Autodesk Inventor part; units mm, degrees
ref_plane "YZ Plane" through (0, 0, 0) normal (1, 0, 0) x (0, 1, 0)
ref_plane "XZ Plane" through (0, 0, 0) normal (0, 1, 0) x (-1, 0, 0)
ref_plane "XY Plane" through (0, 0, 0) normal (0, 0, 1) x (1, 0, 0)
sketch "スケッチ2" plane through (0, 0, 0) normal (0, 1, 0) x (-1, 0, 0)
  circle A0 centre (0, 0) radius 2
  circle A1 centre (0, 0) radius 2.75
  circle A2 centre (0, 0) radius 3.5
  line L0 (3.2709, 0) -> (-4.3069, 0) construction
  line L1 (-3.5, -2.0207) -> (0, -4.0415)
  line L2 (-3.5, 0) -> (-3.5, -2.0207)
  line L3 (0, 3.4516) -> (0, -4.8702) construction
  line L4 (-3.5, 2.0207) -> (0, 4.0415)
  line L5 (-3.5, 0) -> (-3.5, 2.0207)
  line L6 (3.5, -2.0207) -> (0, -4.0415)
  line L7 (3.5, 0) -> (3.5, -2.0207)
  line L8 (3.5, 2.0207) -> (0, 4.0415)
  line L9 (3.5, 0) -> (3.5, 2.0207)
  dimension "d8" = 7
  dimension "d6" = 4
  dimension "d7" = 5.5
  dimension "d25" = 120
extrude "押し出し1" add sketch "スケッチ2" against normal blind 0.7 contours A1
extrude "押し出し2" add sketch "スケッチ2" along normal blind 2.1 contours A1 | A2 | L7 L6 A2 | A2 L8 L9 | A2 L4 L8 | L6 L1 A2 | A2 L5 L4 | L1 L2 A2
chamfer "面取り1" distance 0.2 angle 45 6 edges at (3.5, 1.05, -2.0207) (0, 1.05, -4.0415) (-3.5, 1.05, -2.0207) (-3.5, 1.05, 2.0207) (0, 1.05, 4.0415) (3.5, 1.05, 2.0207)
chamfer "面取り2" distance 0.2 angle 45 6 edges at (3.4134, 2.1, -1.9707) (0, 2.1, -3.9415) (-3.4134, 2.1, -1.9707) (-3.4134, 2.1, 1.9707) (0, 2.1, 3.9415) (3.4134, 2.1, 1.9707)
thread "ねじ1"
properties part number "S4-07-3W" material "ステンレス鋼 AISI 304"
Verification items for the finished model (mm, model axes). A direction names the side the tool comes from. Give positions to 0.01 mm unless a question says otherwise; leave off trailing zeros. Loops run counter-clockwise (first coordinate to the right, second up) from the corner with the lowest first, then second, coordinate; pieces in that order, holes last.
1) Sectioned sample at C-C, the plane x = -2.25. Enter the section's corners in (y, z).
2) Sectioned sample at D-D, the plane z = -2.5. Enter the section's corners in (x, y).
3) Sectioned sample at B-B, the plane x = 0. Enter the section's corners in (y, z), then the cut area to 3 significant figures.
4) Draft check along Z on faces 1 (the cylindrical face through (0.596, -0.345, -2.685)), 2 (the cylindrical face through (0, 1, 2)), 3 (the flat face through (-2, 2.1, 2)). Enter one of: pulls with the +Z half, pulls with the -Z half, needs draft (parallel to the pull), parting line crosses it, or undercut.
5) Set-up check for faces 4 (the flat face through (1, 0, 3)), 5 (the flat face through (-1, -0.7, -2)): record each of +Z, -Z, +X, -X, +Y, -Y from which the full face is reachable in a straight line by a thin tool's end or side.
6) Thickness scan on line 1 along Z through (x, y) = (0, 1); line 2 along Z through (x, y) = (-1.5, 1.55); line 3 along Y through (x, z) = (-3, -2). Record the ranges inside material, lowest first.
7) Sectioned sample at A-A, the plane z = 0. Enter the section's corners in (x, y).
8) Depth check by flat-ended pin: pin 1 Ø2 at (x, z) = (1, -1) entering from -Y. Enter the tip coordinate at first touch or a pass-through.
Answers:
1. outline: (-0.7, -1.58) - (0, -1.58) - (0, -2.74) - (2.1, -2.74) - (2.1, 2.74) - (0, 2.74) - (0, 1.58) - (-0.7, 1.58) - close
2. outline: (-2.67, 0) - (-1.15, 0) - (-1.15, -0.7) - (1.15, -0.7) - (1.15, 0) - (2.67, 0) - (2.67, 2.1) - (-2.67, 2.1) - close
3. outline: (-0.7, -2.75) - (0, -2.75) - (0, -3.94) - (1.9, -3.94) - (2.1, -3.74) - (2.1, -2) - (-0.7, -2) - close; (-0.7, 2) - (2.1, 2) - (2.1, 3.74) - (1.9, 3.94) - (0, 3.94) - (0, 2.75) - (-0.7, 2.75) - close
3. area: 9.16 mm2
4. face 1: parting line crosses it
4. face 2: undercut
4. face 3: needs draft
5. face 4: -Y
5. face 5: +Z, -Z, +X, -X, -Y
6. line 1: z = -3.94 to -2, 2 to 3.94
6. line 2: z = -3.18 to -1.32, 1.32 to 3.18
6. line 3: y = 0 to 2.1
7. outline: (-3.5, 0) - (-2.75, 0) - (-2.75, -0.7) - (-2, -0.7) - (-2, 2.1) - (-3.5, 2.1) - close; (2, -0.7) - (2.75, -0.7) - (2.75, 0) - (3.5, 0) - (3.5, 2.1) - (2, 2.1) - close
8. pin 1: stops at y = -0.7
